The figure shows three views and two pictorial views of one solid part (mm, origin at its lowest corner). Answer the questions. A direction names the side the tool comes from. Give positions to 0.01 mm unless a question says otherwise; leave off trailing zeros. Order: outer loops, then holes, each group sorted by start corner. A loop starts at its lowest first (then second) coordinate and runs counter-clockwise, first axis right, second up. Notation, with made-up numbers: (2, 50) - (26, 50) arc R11 ccw to (26, 59) - close; hole circle Ø10 at (44, 80). An arc over 180 degrees is marked (long way). Answer as a JSON object with one key per item and string values. Group by question number.
Q1. A cutting plane is placed at D-D, the plane z = 33. Give the vertices of the cut face in (x, y), and give its area (3 significant figures).
Q2. Consider line 1 (X direction, y = 2.85, z = 18.5) (1 decimal); line 2 (Z direction, x = 13.25, y = 3.05); line 3 (Z direction, x = 13.25, y = 1.15). Determine where each line is inside the solid, lowest interval first.
Q3. A cutting plane is placed at A-A, the plane y = 3. Count the separate pieces of the cut face and the enclosed holes in it.
Q4. A cutting plane is placed at B-B, the plane z = 18.5. Give the vertices of the cut face in (x, y) (1 decimal).
Q5. The mould has two halves that part along Z. Classify the marked faces 1, 2, 3 and 4: released by +Z, released by -Z, zero draft, split by the parting line, or undercut.
Q6. For the marked faces 5, 6, 7 and 8, determine the directions among +Z, -Z, +X, -X, +Y, -Y from which every point of the face is accessible in a straight line to the end or side of a thin tool.
Q7. A cutting plane is placed at C-C, the plane x = 10. Give the vertices of the cut face in (y, z), and give its area (3 significant figures).
Q8. Given pin 1 (1.8 mm diameter, centred on x = 27.5, y = 3, fed in from +Z); pin 2 (3.5 mm diameter, centred on y = 2.5, z = 8, fed in from -X); pin 3 (1 mm diameter, centred on x = 10, y = 1, fed in from -Z); pin 4 (3.5 mm diameter, centred on y = 4.5, z = 9, fed in from +X) (1 decimal), each flat-ended and moving along its own axis, determine where each tip first touches the part or whether it passes through.
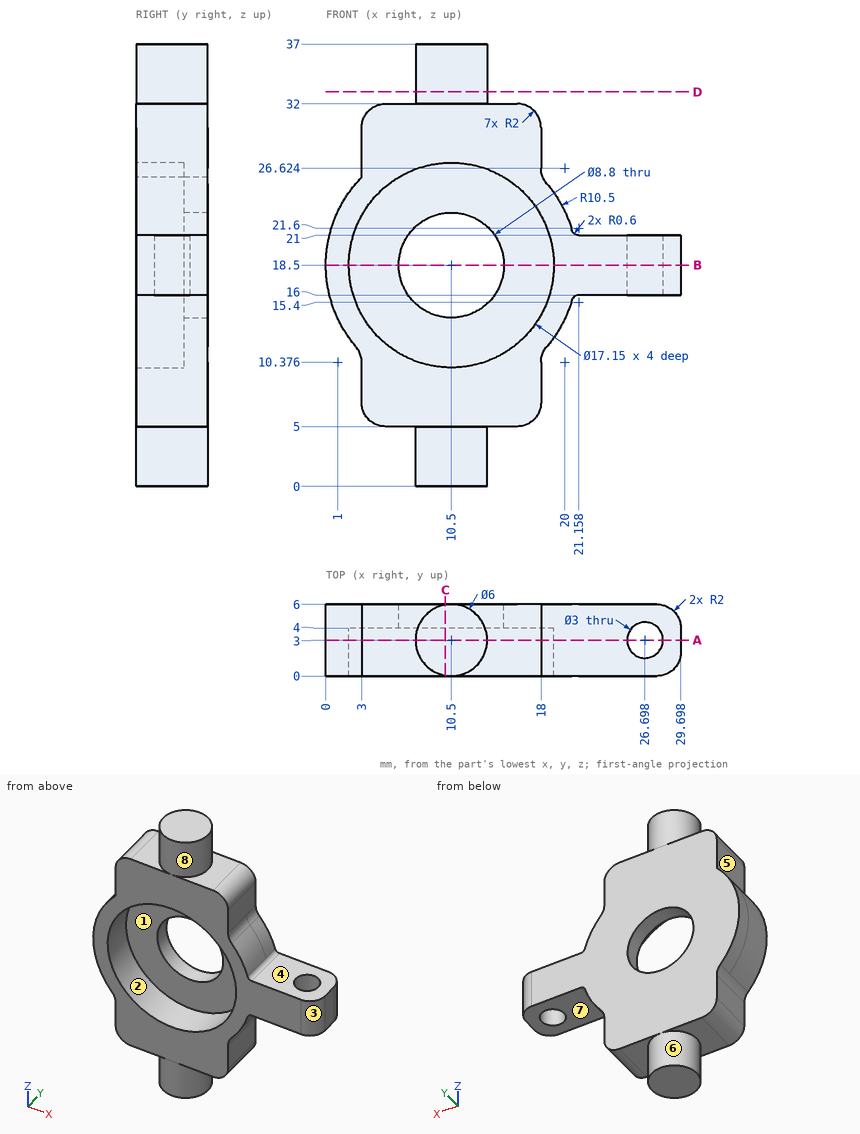
Reply:
{
 "1": {"outline": "circle Ø6 at (10.5, 3)", "area": "28.3 mm^2"},
 "2": {"line 1": "x = 0 to 1.9, 19.1 to 25.2, 28.2 to 29.7", "line 2": "z = 0 to 10.38, 26.62 to 37", "line 3": "z = 5 to 10.38, 26.62 to 32"},
 "3": {"separate pieces": "2", "enclosed holes": "1"},
 "4": {"outline": "(0, 0) - (1.9, 0) - (1.9, 4) - (6.1, 4) - (6.1, 6) - (0, 6) - close; (14.9, 4) - (19.1, 4) - (19.1, 0) - (27.7, 0) arc R2 ccw to (29.7, 2) - (29.7, 4) arc R2 ccw to (27.7, 6) - (14.9, 6) - close; hole circle Ø3 at (26.7, 3)"},
 "5": {"face 1": "undercut", "face 2": "undercut", "face 3": "zero draft", "face 4": "released by +Z"},
 "6": {"face 5": "+Z, -X, +Y, -Y", "face 6": "-Z", "face 7": "-Z, +X, +Y, -Y", "face 8": "+Z"},
 "7": {"outline": "(0, 5) - (0.04, 5) - (0.04, 0) - (5.96, 0) - (5.96, 5) - (6, 5) - (6, 14.13) - (4, 14.13) - (4, 9.94) - (0, 9.94) - close; (0, 27.06) - (4, 27.06) - (4, 22.87) - (6, 22.87) - (6, 32) - (5.96, 32) - (5.96, 37) - (0.04, 37) - (0.04, 32) - (0, 32) - close", "area": "135 mm^2"},
 "8": {"pin 1": "stops at z = 21", "pin 2": "stops at x = 3", "pin 3": "stops at z = 0", "pin 4": "stops at x = 18"}
}
